Build history of the part. All positions in model axes, mm. Face numbers are marked on the shaded views. A direction names the side the tool comes from. Coordinates: 2 decimals unless noted, no trailing zeros. Order: outer loops, then holes, each group sorted by start corner. A loop starts at its lowest first (then second) coordinate and runs counter-clockwise, first axis right, second up. Notation, with made-up numbers: M 79,-4.5 L 133,-4.5 A19 cw 133,18.5 Z; hole C -28.75,-12.75 d11. An arc over 180 degrees is marked long. Write item = value, one per line. Start each with the question number.
Q1. Drill centre lines: probe 1 along Z at (x, y) = (8.75, 0); probe 2 along Y at (x, z) = (12, 18); probe 3 along Z at (x, y) = (11, -18). Where is each one in solid material? Low to high.
Q2. Pin check, flat tips, straight feed: P1, Ø1, axis at x = 12.5, z = -17, coming from the -Y side; P2, Ø3, axis at x = 14.5, y = -3, coming from the +Z side; P3, Ø3, axis at x = 11.5, y = -11.5, coming from the +Z side; P4, Ø4, axis at x = 10.5, z = -15.5, coming from the -Y side. Stop position of each tip, or through.
Q3. Pull direction Y, two halves, no side cores. Call the marked faces 1, 2 and 3: released by +Y, released by -Y, zero draft, split by the parting line, or undercut.
Q4. Band-saw the part on A-A on y = 0. Write the cut outline in (x, z), plus the area to 3 significant figures.
Q5. 3-axis set-ups, long thin cutter, end or side, ignore diameter. For the marked faces 4, 5, 6 and 7: which of +Z, -Z, +X, -X, +Y, -Y reach the whole face in a straight line?
```python
from build123d import *

# Parameters (mm, degrees)
BASPROSKE_W         = 15
BASPROSKE_H         = 22
TOOTHCUT_DEPTH      = 35.539832078
TEETHCUTS_COUNT     = 20
TEETHCUTS_ANGLE     = 342
BORSKE_R            = 0.5
BORE_DEPTH          = 50.0000508
SKETCH1_R           = 11.1
CUT_EXTRUDE1_DEPTH  = 16
CUT_EXTRUDE2_DEPTH  = 8
SKETCH3_R           = 11.1
BOSS_EXTRUDE1_DEPTH = 7
CUT_EXTRUDE3_DEPTH  = 7
SKETCH5_R           = 17.499
BOSS_EXTRUDE2_DEPTH = 7


with BuildPart() as part:
    # BasProSke → Base-Revolve (revolve)
    with BuildSketch(Plane(origin=(0, 0, 0), x_dir=(1, 0, 0), z_dir=(0, 1, 0)), mode=Mode.PRIVATE) as base_revolve_sk:
        with Locations((7.5, 11)):
            Rectangle(BASPROSKE_W, BASPROSKE_H)
    revolve(base_revolve_sk.sketch.rotate(Axis((-10, 0, 0), (1, 0, 0)), 180), axis=Axis((-10, 0, 0), (1, 0, 0)))

    # TooCutSke → ToothCut (cut, through all)
    with BuildSketch(Plane(origin=(0, 0, 0), x_dir=(0, 0, -1), z_dir=(1, 0, 0))):
        with BuildLine():
            ThreePointArc((0.986171591, 17.471189616), (0, 17.499), (-0.986171591, 17.471189616))
            ThreePointArc((-0.986171591, 17.471189616), (-1.626916196, 19.798789858), (-2.932850173, 21.829260982))
            ThreePointArc((-2.932850173, 21.829260982), (0, 22.0254), (2.932850173, 21.829260982))
            ThreePointArc((2.932850173, 21.829260982), (1.626916196, 19.798789858), (0.986171591, 17.471189616))
        make_face()
    toothcut = extrude(amount=TOOTHCUT_DEPTH, mode=Mode.SUBTRACT)

    # TeethCuts: ToothCut ×20 about axis
    teethcuts_axis = Axis((-10, 0, 0), (1, 0, 0))
    for i in range(1, TEETHCUTS_COUNT):
        add(toothcut.rotate(teethcuts_axis, i * TEETHCUTS_ANGLE / (TEETHCUTS_COUNT - 1)), mode=Mode.SUBTRACT)

    # BorSke → Bore (cut, symmetric)
    with BuildSketch(Plane(origin=(0, 0, 0), x_dir=(0, 0, -1), z_dir=(1, 0, 0))):
        with Locations(Location((0, 0, 0), (0, 0, 180))):
            Circle(BORSKE_R)
    extrude(amount=BORE_DEPTH, both=True, mode=Mode.SUBTRACT)

    # Sketch1 → Cut-Extrude1 (cut)
    with BuildSketch(Plane.ZY):
        Circle(SKETCH1_R)
    extrude(amount=-CUT_EXTRUDE1_DEPTH, mode=Mode.SUBTRACT)

    # Sketch2 → Cut-Extrude2 (cut)
    with BuildSketch(Plane.ZY):
        with BuildLine():
            ThreePointArc((17.471189616, 0.986171591), (19.784848102, 1.620704589), (21.806333941, 2.912696354))
            ThreePointArc((21.806333941, 2.912696354), (21.729143493, 3.441558231), (21.639128664, 3.968388926))
            ThreePointArc((21.639128664, 3.968388926), (19.317333972, 4.572472634), (16.920832513, 4.460989585))
            ThreePointArc((16.920832513, 4.460989585), (16.642537979, 5.407488385), (16.31134495, 6.336799421))
            ThreePointArc((16.31134495, 6.336799421), (18.31568345, 7.655235955), (19.838983319, 9.50866662))
            ThreePointArc((19.838983319, 9.50866662), (19.602143532, 9.987790994), (19.353734704, 10.461020648))
            ThreePointArc((19.353734704, 10.461020648), (16.958904602, 10.318064378), (14.714146429, 9.471478019))
            ThreePointArc((14.714146429, 9.471478019), (14.156988385, 10.28565413), (13.554832194, 11.067137173))
            ThreePointArc((13.554832194, 11.067137173), (15.05365209, 12.940419489), (15.929654782, 15.173862347))
            ThreePointArc((15.929654782, 15.173862347), (15.556349186, 15.556349186), (15.173862347, 15.929654782))
            ThreePointArc((15.173862347, 15.929654782), (12.940419489, 15.05365209), (11.067137173, 13.554832194))
            ThreePointArc((11.067137173, 13.554832194), (10.28565413, 14.156988385), (9.471478019, 14.714146429))
            ThreePointArc((9.471478019, 14.714146429), (10.318064378, 16.958904602), (10.461020648, 19.353734704))
            ThreePointArc((10.461020648, 19.353734704), (9.987790994, 19.602143532), (9.50866662, 19.838983319))
            ThreePointArc((9.50866662, 19.838983319), (7.655235955, 18.31568345), (6.336799421, 16.31134495))
            ThreePointArc((6.336799421, 16.31134495), (5.407488385, 16.642537979), (4.460989585, 16.920832513))
            ThreePointArc((4.460989585, 16.920832513), (4.572472634, 19.317333972), (3.968388926, 21.639128664))
            ThreePointArc((3.968388926, 21.639128664), (3.441558231, 21.729143493), (2.912696354, 21.806333941))
            ThreePointArc((2.912696354, 21.806333941), (1.620704589, 19.784848102), (0.986171591, 17.471189616))
            ThreePointArc((0.986171591, 17.471189616), (0, 17.499), (-0.986171591, 17.471189616))
            ThreePointArc((-0.986171591, 17.471189616), (-1.620704589, 19.784848102), (-2.912696354, 21.806333941))
            ThreePointArc((-2.912696354, 21.806333941), (-3.441558231, 21.729143493), (-3.968388926, 21.639128664))
            ThreePointArc((-3.968388926, 21.639128664), (-4.572472634, 19.317333972), (-4.460989585, 16.920832513))
            ThreePointArc((-4.460989585, 16.920832513), (-5.407488385, 16.642537979), (-6.336799421, 16.31134495))
            ThreePointArc((-6.336799421, 16.31134495), (-7.655235955, 18.31568345), (-9.50866662, 19.838983319))
            ThreePointArc((-9.50866662, 19.838983319), (-9.987790994, 19.602143532), (-10.461020648, 19.353734704))
            ThreePointArc((-10.461020648, 19.353734704), (-10.318064378, 16.958904602), (-9.471478019, 14.714146429))
            ThreePointArc((-9.471478019, 14.714146429), (-10.28565413, 14.156988385), (-11.067137173, 13.554832194))
            ThreePointArc((-11.067137173, 13.554832194), (-12.940419489, 15.05365209), (-15.173862347, 15.929654782))
            ThreePointArc((-15.173862347, 15.929654782), (-15.556349186, 15.556349186), (-15.929654782, 15.173862347))
            ThreePointArc((-15.929654782, 15.173862347), (-15.05365209, 12.940419489), (-13.554832194, 11.067137173))
            ThreePointArc((-13.554832194, 11.067137173), (-14.156988385, 10.28565413), (-14.714146429, 9.471478019))
            ThreePointArc((-14.714146429, 9.471478019), (-16.958904602, 10.318064378), (-19.353734704, 10.461020648))
            ThreePointArc((-19.353734704, 10.461020648), (-19.602143532, 9.987790994), (-19.838983319, 9.50866662))
            ThreePointArc((-19.838983319, 9.50866662), (-18.31568345, 7.655235955), (-16.31134495, 6.336799421))
            ThreePointArc((-16.31134495, 6.336799421), (-16.642537979, 5.407488385), (-16.920832513, 4.460989585))
            ThreePointArc((-16.920832513, 4.460989585), (-19.317333972, 4.572472634), (-21.639128664, 3.968388926))
            ThreePointArc((-21.639128664, 3.968388926), (-21.729143493, 3.441558231), (-21.806333941, 2.912696354))
            ThreePointArc((-21.806333941, 2.912696354), (-19.784848102, 1.620704589), (-17.471189616, 0.986171591))
            ThreePointArc((-17.471189616, 0.986171591), (-17.499, 0), (-17.471189616, -0.986171591))
            ThreePointArc((-17.471189616, -0.986171591), (-19.784848102, -1.620704589), (-21.806333941, -2.912696354))
            ThreePointArc((-21.806333941, -2.912696354), (-21.729143493, -3.441558231), (-21.639128664, -3.968388926))
            ThreePointArc((-21.639128664, -3.968388926), (-19.317333972, -4.572472634), (-16.920832513, -4.460989585))
            ThreePointArc((-16.920832513, -4.460989585), (-16.642537979, -5.407488385), (-16.31134495, -6.336799421))
            ThreePointArc((-16.31134495, -6.336799421), (-18.31568345, -7.655235955), (-19.838983319, -9.50866662))
            ThreePointArc((-19.838983319, -9.50866662), (-19.602143532, -9.987790994), (-19.353734704, -10.461020648))
            ThreePointArc((-19.353734704, -10.461020648), (-16.958904602, -10.318064378), (-14.714146429, -9.471478019))
            ThreePointArc((-14.714146429, -9.471478019), (-14.156988385, -10.28565413), (-13.554832194, -11.067137173))
            ThreePointArc((-13.554832194, -11.067137173), (-15.05365209, -12.940419489), (-15.929654782, -15.173862347))
            ThreePointArc((-15.929654782, -15.173862347), (-15.556349186, -15.556349186), (-15.173862347, -15.929654782))
            ThreePointArc((-15.173862347, -15.929654782), (-12.940419489, -15.05365209), (-11.067137173, -13.554832194))
            ThreePointArc((-11.067137173, -13.554832194), (-10.28565413, -14.156988385), (-9.471478019, -14.714146429))
            ThreePointArc((-9.471478019, -14.714146429), (-10.318064378, -16.958904602), (-10.461020648, -19.353734704))
            ThreePointArc((-10.461020648, -19.353734704), (-9.987790994, -19.602143532), (-9.50866662, -19.838983319))
            ThreePointArc((-9.50866662, -19.838983319), (-7.655235955, -18.31568345), (-6.336799421, -16.31134495))
            ThreePointArc((-6.336799421, -16.31134495), (-5.407488385, -16.642537979), (-4.460989585, -16.920832513))
            ThreePointArc((-4.460989585, -16.920832513), (-4.572472634, -19.317333972), (-3.968388926, -21.639128664))
            ThreePointArc((-3.968388926, -21.639128664), (-3.441558231, -21.729143493), (-2.912696354, -21.806333941))
            ThreePointArc((-2.912696354, -21.806333941), (-1.620704589, -19.784848102), (-0.986171591, -17.471189616))
            ThreePointArc((-0.986171591, -17.471189616), (0, -17.499), (0.986171591, -17.471189616))
            ThreePointArc((0.986171591, -17.471189616), (1.620704589, -19.784848102), (2.912696354, -21.806333941))
            ThreePointArc((2.912696354, -21.806333941), (3.441558231, -21.729143493), (3.968388926, -21.639128664))
            ThreePointArc((3.968388926, -21.639128664), (4.572472634, -19.317333972), (4.460989585, -16.920832513))
            ThreePointArc((4.460989585, -16.920832513), (5.407488385, -16.642537979), (6.336799421, -16.31134495))
            ThreePointArc((6.336799421, -16.31134495), (7.655235955, -18.31568345), (9.50866662, -19.838983319))
            ThreePointArc((9.50866662, -19.838983319), (9.987790994, -19.602143532), (10.461020648, -19.353734704))
            ThreePointArc((10.461020648, -19.353734704), (10.318064378, -16.958904602), (9.471478019, -14.714146429))
            ThreePointArc((9.471478019, -14.714146429), (10.28565413, -14.156988385), (11.067137173, -13.554832194))
            ThreePointArc((11.067137173, -13.554832194), (12.940419489, -15.05365209), (15.173862347, -15.929654782))
            ThreePointArc((15.173862347, -15.929654782), (15.556349186, -15.556349186), (15.929654782, -15.173862347))
            ThreePointArc((15.929654782, -15.173862347), (15.05365209, -12.940419489), (13.554832194, -11.067137173))
            ThreePointArc((13.554832194, -11.067137173), (14.156988385, -10.28565413), (14.714146429, -9.471478019))
            ThreePointArc((14.714146429, -9.471478019), (16.958904602, -10.318064378), (19.353734704, -10.461020648))
            ThreePointArc((19.353734704, -10.461020648), (19.602143532, -9.987790994), (19.838983319, -9.50866662))
            ThreePointArc((19.838983319, -9.50866662), (18.31568345, -7.655235955), (16.31134495, -6.336799421))
            ThreePointArc((16.31134495, -6.336799421), (16.642537979, -5.407488385), (16.920832513, -4.460989585))
            ThreePointArc((16.920832513, -4.460989585), (19.317333972, -4.572472634), (21.639128664, -3.968388926))
            ThreePointArc((21.639128664, -3.968388926), (21.729143493, -3.441558231), (21.806333941, -2.912696354))
            ThreePointArc((21.806333941, -2.912696354), (19.784848102, -1.620704589), (17.471189616, -0.986171591))
            ThreePointArc((17.471189616, -0.986171591), (17.499, 0), (17.471189616, 0.986171591))
        make_face()
    extrude(amount=-CUT_EXTRUDE2_DEPTH, mode=Mode.SUBTRACT)

    # Sketch3 → Boss-Extrude1 (add)
    with BuildSketch(Plane.ZY.offset(-8)):
        Circle(SKETCH3_R)
    extrude(amount=-BOSS_EXTRUDE1_DEPTH)

    # Sketch4 → Cut-Extrude3 (cut)
    with BuildSketch(Plane.ZY.offset(-8)):
        Polygon((21.729143493, -3.441558231), (0, 0), (-21.729143493, 3.441558231), (-17.979863548, 27.113580164), (25.478423438, 20.230463702), align=None)
    extrude(amount=-CUT_EXTRUDE3_DEPTH, mode=Mode.SUBTRACT)

    # Sketch5 → Boss-Extrude2 (add)
    with BuildSketch(Plane.ZY.offset(-8)):
        Circle(SKETCH5_R)
    extrude(amount=-BOSS_EXTRUDE2_DEPTH)


solid = part.part
```
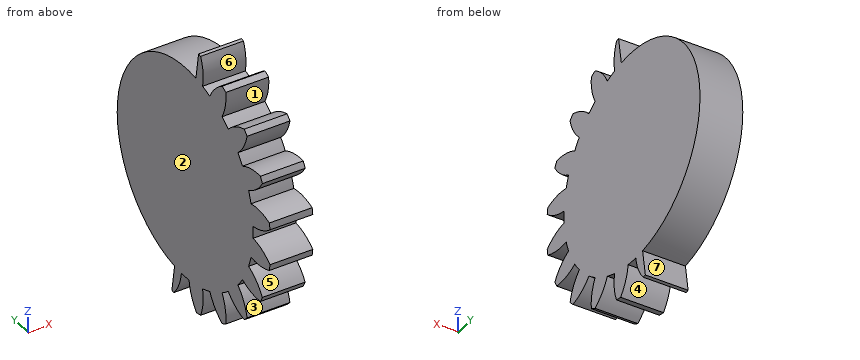
Recorded:
q1.probe_1 = -17.5 to 17.5
q1.probe_2 = -10.47 to -7.39, -4.6 to -2.85
q1.probe_3 = -10.47 to -7.39, -4.6 to -1.07, 1.07 to 4.6, 7.39 to 10.47
q2.P1 = -10.41
q2.P2 = 21.73
q2.P3 = 19.6
q2.P4 = -15.93
q3.face_1 = undercut
q3.face_2 = zero draft
q3.face_3 = released by -Y
q4.outline = M 8,-17.5 L 15,-17.5 L 15,17.5 L 8,17.5 Z
q4.area = 245 mm2
q5.face_4 = -Z, +X, -X
q5.face_5 = +X, -X, -Y
q5.face_6 = +X, -X
q5.face_7 = +X, -X, +Y
